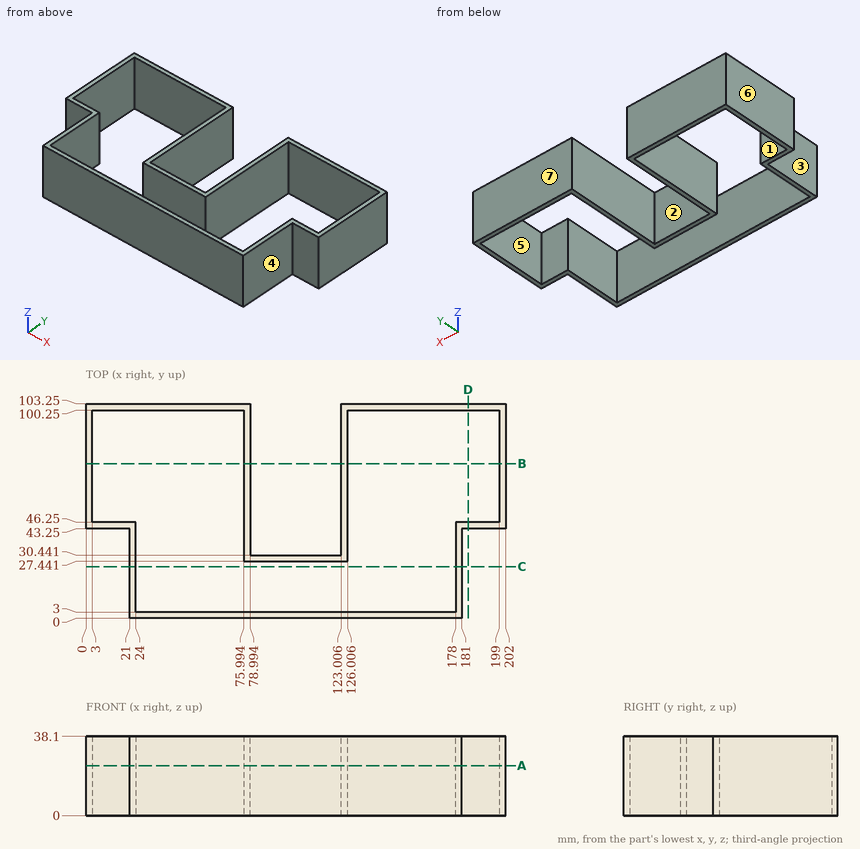
Geometry check sheet. Reference: drawing and pictorial views, mm from the part's lowest x, y, z. A direction names the side the tool comes from. Give positions to 0.01 mm unless a question says otherwise; leave off trailing zeros. Loops run counter-clockwise (first coordinate to the right, second up) from the corner with the lowest first, then second, coordinate; pieces in that order, holes last. Notation, with made-up numbers: (46, 55) - (74, 55) arc R32 ccw to (74, 84) - close; hole circle Ø7 at (68, 56). An arc over 180 degrees is marked (long way). Use CSV: the item, a comma, the result in double quotes. Start each with the question number.
Q1. Section check D-D, the plane x = 184. Record the cut outline in (y, z).
Q2. Scan lines: probe 1 along X at (y, z) = (66, 11); probe 2 along X at (y, z) = (35.5, 23.5); probe 3 along Y at (x, z) = (146, 21). Record each from-to range of solid material in increasing order. Write a range as from..to.
Q3. Access from +Z, -Z, +X, -X, +Y, -Y to the whole of each face (thin tool, end or side, straight path). Record for the marked faces 1, 2, 3 and 4.
Q4. Go/stop test with flat-tipped pins: pin 1 Ø1.5 at (y, z) = (40, 9.5) entering from -X; pin 2 Ø10.5 at (x, z) = (189.5, 27.5) entering from -Y; pin 3 Ø11.5 at (x, z) = (101.5, 15.5) entering from +Y. Record where each tip stops, or that it passes through.
Q5. Section check B-B, the plane y = 74.5. Record the cut outline in (x, z).
Q6. Section check A-A, the plane z = 24. Record the cut outline in (x, y), and give its area (3 significant figures).
Q7. Section check C-C, the plane y = 25. Record the cut outline in (x, z).
Q8. Release check for a two-part mould opening along X. For the marked faces 5, 6 and 7 record: +X half, -X half, draft (parallel to the pull), parting line (faces both ways), or undercut.
Findings below:
1,outline,"(43.25, 0) - (46.25, 0) - (46.25, 38.1) - (43.25, 38.1) - close; (100.25, 0) - (103.25, 0) - (103.25, 38.1) - (100.25, 38.1) - close"
2,probe 1,"x = 0..3, 75.99..78.99, 123.01..126.01, 199..202"
2,probe 2,"x = 21..24, 75.99..78.99, 123.01..126.01, 178..181"
2,probe 3,"y = 0..3, 100.25..103.25"
3,face 1,"+Z, -Z"
3,face 2,"+Z, -Z, +Y"
3,face 3,"+Z, -Z, -X, -Y"
3,face 4,"+Z, -Z, +X, -Y"
4,pin 1,"stops at x = 21"
4,pin 2,"stops at y = 43.25"
4,pin 3,"stops at y = 30.44"
5,outline,"(0, 0) - (3, 0) - (3, 38.1) - (0, 38.1) - close; (75.99, 0) - (78.99, 0) - (78.99, 38.1) - (75.99, 38.1) - close; (123.01, 0) - (126.01, 0) - (126.01, 38.1) - (123.01, 38.1) - close; (199, 0) - (202, 0) - (202, 38.1) - (199, 38.1) - close"
6,outline,"(0, 43.25) - (21, 43.25) - (21, 0) - (181, 0) - (181, 43.25) - (202, 43.25) - (202, 103.25) - (123.01, 103.25) - (123.01, 30.44) - (78.99, 30.44) - (78.99, 103.25) - (0, 103.25) - close; hole (3, 46.25) - (24, 46.25) - (24, 3) - (178, 3) - (178, 46.25) - (199, 46.25) - (199, 100.25) - (126.01, 100.25) - (126.01, 27.44) - (75.99, 27.44) - (75.99, 100.25) - (3, 100.25) - close"
6,area,"2,230 mm^2"
7,outline,"(21, 0) - (24, 0) - (24, 38.1) - (21, 38.1) - close; (178, 0) - (181, 0) - (181, 38.1) - (178, 38.1) - close"
8,face 5,"undercut"
8,face 6,"-X half"
8,face 7,"draft"
